```python
from build123d import *

# Parameters (mm, degrees)
F1_DEPTH = 25.4
F2_T     = -2.54


with BuildPart() as f1:
    # F0 (on Front) → F1 (new body)
    with BuildSketch(Plane.XZ):
        Polygon((0, 25.4), (0, 0), (25.4, 0), (25.4, 20.32), (22.86, 20.32), (22.86, 22.86), (25.4, 22.86), (25.4, 25.4), align=None)
    extrude(amount=F1_DEPTH)

    # F2
    f2_openings = [f1.faces().sort_by_distance(p)[0] for p in [
        (25.4, -12.7, 10.16),
    ]]
    offset(amount=F2_T, openings=f2_openings, kind=Kind.INTERSECTION)


solid = f1.part
```
For this review, take the finished solid that the model builds, in its own axes (mm). A direction names the side the tool comes from. Give positions to 0.01 mm unless a question says otherwise; leave off trailing zeros. Write each loop counter-clockwise with the first axis right and the second up, starting at its lowest first coordinate (ties: lowest second). Pieces come first, ordered by that corner, then holes.
Item 1: The part is to be moulded in two halves that separate along X. For faces 1 (the face through (0, -13, 13)), 2 (the face through (13, -13, 0)), 3 (the face through (25.4, -13, 1)), 4 (the face through (20.32, -13, 20)), say which applies: +X half, -X half, draft (parallel to the pull), parting line (faces both ways), or undercut.
Item 2: Insertion check: P1, Ø2, axis at y = -14.5, z = 21.5, coming from the +X side; P2, Ø2, axis at y = -12.5, z = 10.5, coming from the +X side. Each pin has a flat end and moves straight along its axis. Give the tip position at first contact, or say it passes through.
Item 3: Take a section at B-B (x = 4.25). Give the boundary of the cut face in (y, z), and give its area (3 significant figures).
Item 4: Take a section at D-D (z = 12.25). Give the boundary of the cut face in (x, y), and give its area (3 significant figures).
Item 5: Machinability: for faces 5 (the face through (23, -13, 17.78)), 6 (the face through (22.86, -13, 22)), 7 (the face through (14, -2.54, 13)), 8 (the face through (13, -25.4, 13)), which of the approach directions +Z, -Z, +X, -X, +Y, -Y give a long, thin tool a straight path to every point of the face, cutting with its end or side? Answer none if there is none.
Item 6: Wall thickness on probe 1 along Z at (x, y) = (24.25, -11); probe 2 along Y at (x, z) = (8.5, 18.5); probe 3 along X at (y, z) = (-13, 20): over which ranges is each line inside the solid? List them lowest first.
Item 7: Take a section at A-A (z = 22.25). Give the boundary of the cut face in (x, y).
Item 8: Take a section at C-C (y = -7.5). Give the boundary of the cut face in (x, z), and give its area (3 significant figures).
Established:
1. face 1: -X half
1. face 2: draft
1. face 3: +X half
1. face 4: undercut
2. P1: stops at x = 22.86
2. P2: stops at x = 2.54
3. outline: (-25.4, 0) - (0, 0) - (0, 25.4) - (-25.4, 25.4) - close; hole (-22.86, 2.54) - (-2.54, 2.54) - (-2.54, 22.86) - (-22.86, 22.86) - close
3. area: 232 mm2
4. outline: (0, -25.4) - (25.4, -25.4) - (25.4, -22.86) - (2.54, -22.86) - (2.54, -2.54) - (25.4, -2.54) - (25.4, 0) - (0, 0) - close
4. area: 181 mm2
5. face 5: +X
5. face 6: +X, +Y, -Y
5. face 7: none
5. face 8: +Z, -Z, +X, -X, -Y
6. probe 1: z = 0 to 2.54, 17.78 to 20.32, 22.86 to 25.4
6. probe 2: y = -25.4 to -22.86, -2.54 to 0
6. probe 3: x = 0 to 2.54, 20.32 to 25.4
7. outline: (0, -25.4) - (22.86, -25.4) - (22.86, 0) - (0, 0) - close; hole (2.54, -22.86) - (20.32, -22.86) - (20.32, -2.54) - (2.54, -2.54) - close
8. outline: (0, 0) - (25.4, 0) - (25.4, 2.54) - (2.54, 2.54) - (2.54, 22.86) - (20.32, 22.86) - (20.32, 17.78) - (25.4, 17.78) - (25.4, 20.32) - (22.86, 20.32) - (22.86, 22.86) - (25.4, 22.86) - (25.4, 25.4) - (0, 25.4) - close
8. area: 200 mm2
